Here's how the part is built. I have some questions about the finished solid (model axes, mm). A direction names the side the tool comes from. Coordinates: 2 decimals unless noted, no trailing zeros. Answer as a JSON object with one key per item and string values. Group by question number.
Q1. On a 3-axis mill with a long thin cutter (end or side, diameter ignored), from which of +Z, -Z, +X, -X, +Y, -Y can I reach the whole of each face in a straight line? I mean faces 4 (the flat face through (4, 200, 0)), 5 (the flat face through (0, 99, 4.5)). Say none if no direction works.
Q2. I need wall thicknesses on line 1 (Z direction, x = 8, y = 101.5); line 2 (Z direction, x = 3.75, y = 88.5). Which ranges of each line are inside material? Lowest first, please.
Q3. I'm going to push flat-ended pins straight in: pin 1 (0.6 mm diameter, centred on y = 59.5, z = 10, fed in from +X); pin 2 (0.6 mm diameter, centred on x = 9.5, y = 65, fed in from +Z); pin 3 (1.5 mm diameter, centred on x = -1, z = -0.5, fed in from -Y); pin 4 (2 mm diameter, centred on y = 113.5, z = 1.5, fed in from -X). Where does each tip first touch, or does it pass through?
Q4. Thinking about a two-plate mould opening in X: for faces 1 (the flat face through (10, 99, -6)), 2 (the flat face through (4, 0, 0)), 3 (the flat face through (0, 99, -4.5)), which applies, released by +X, released by -X, zero draft, split by the parting line, or undercut?
```python
from build123d import *

# Parameters (mm, degrees)
DODANIE_WYCI_GNI_CIE1_DEPTH     = 807
SCHNITT_LINEAR_AUSTRAGEN1_DEPTH = 20


with BuildPart() as part:
    # Szkic1 → Dodanie-wyciągnięcie1 (new body)
    with BuildSketch(Plane(origin=(0, 0, 0), x_dir=(1, 0, 0), z_dir=(0, 1, 0))):
        with BuildLine():
            Line((-7.06, 6), (-4.5, 3.440546933))
            Line((-4.5, 3.440546933), (-4.5, 4.5))
            Line((-4.5, 4.5), (-3.440546933, 4.5))
            Line((-3.440546933, 4.5), (-6, 7.06))
            Line((-6, 7.06), (-6, 8.5))
            Line((-6, 8.5), (-3, 8.5))
            Line((-3, 8.5), (-3, 9.5))
            Line((-3, 9.5), (-3.5, 9.5))
            Line((-3.5, 9.5), (-3.5, 10))
            Line((-3.5, 10), (-8.5, 10))
            ThreePointArc((-8.5, 10), (-9.560660172, 9.560660172), (-10, 8.5))
            Line((-10, 8.5), (-10, 3.5))
            Line((-10, 3.5), (-9.5, 3.5))
            Line((-9.5, 3.5), (-9.5, 3))
            Line((-9.5, 3), (-8.5, 3))
            Line((-8.5, 3), (-8.5, 6))
            Line((-8.5, 6), (-7.06, 6))
        make_face()
        with BuildLine():
            Line((4.5, 4.5), (4.5, 3.440546933))
            Line((4.5, 3.440546933), (7.06, 6))
            Line((7.06, 6), (8.5, 6))
            Line((8.5, 6), (8.5, 3))
            Line((8.5, 3), (9.5, 3))
            Line((9.5, 3), (9.5, 3.5))
            Line((9.5, 3.5), (10, 3.5))
            Line((10, 3.5), (10, 8.5))
            ThreePointArc((10, 8.5), (9.560660172, 9.560660172), (8.5, 10))
            Line((8.5, 10), (3.5, 10))
            Line((3.5, 10), (3.5, 9.5))
            Line((3.5, 9.5), (3, 9.5))
            Line((3, 9.5), (3, 8.5))
            Line((3, 8.5), (6, 8.5))
            Line((6, 8.5), (6, 7.06))
            Line((6, 7.06), (3.440546933, 4.5))
            Line((3.440546933, 4.5), (4.5, 4.5))
        make_face()
        Polygon((3.440546933, -4.5), (4.5, -4.5), (4.5, -3.440546933), (4.5, 3.440546933), (4.5, 4.5), (3.440546933, 4.5), (-3.440546933, 4.5), (-4.5, 4.5), (-4.5, 3.440546933), (-4.5, -3.440546933), (-4.5, -4.5), (-3.440546933, -4.5), align=None)
        with BuildLine():
            Line((-3.00520382, 1.944543648), (-1.944543648, 3.00520382))
            Line((-1.944543648, 3.00520382), (-1.271309214, 2.438498079))
            ThreePointArc((-1.271309214, 2.438498079), (0, 2.75), (1.271309214, 2.438498079))
            Line((1.271309214, 2.438498079), (1.944543648, 3.00520382))
            Line((1.944543648, 3.00520382), (3.00520382, 1.944543648))
            Line((3.00520382, 1.944543648), (2.438498079, 1.271309214))
            ThreePointArc((2.438498079, 1.271309214), (2.670989491, 0.654457899), (2.75, 0))
            ThreePointArc((2.75, 0), (2.670989491, -0.654457899), (2.438498079, -1.271309214))
            Line((2.438498079, -1.271309214), (3.00520382, -1.944543648))
            Line((3.00520382, -1.944543648), (1.944543648, -3.00520382))
            Line((1.944543648, -3.00520382), (1.271309214, -2.438498079))
            ThreePointArc((1.271309214, -2.438498079), (0, -2.75), (-1.271309214, -2.438498079))
            Line((-1.271309214, -2.438498079), (-1.944543648, -3.00520382))
            Line((-1.944543648, -3.00520382), (-3.00520382, -1.944543648))
            Line((-3.00520382, -1.944543648), (-2.438498079, -1.271309214))
            ThreePointArc((-2.438498079, -1.271309214), (-2.75, 0), (-2.438498079, 1.271309214))
            Line((-2.438498079, 1.271309214), (-3.00520382, 1.944543648))
        make_face(mode=Mode.SUBTRACT)
        with BuildLine():
            Line((-6, -7.06), (-3.440546933, -4.5))
            Line((-3.440546933, -4.5), (-4.5, -4.5))
            Line((-4.5, -4.5), (-4.5, -3.440546933))
            Line((-4.5, -3.440546933), (-7.06, -6))
            Line((-7.06, -6), (-8.5, -6))
            Line((-8.5, -6), (-8.5, -3))
            Line((-8.5, -3), (-9.5, -3))
            Line((-9.5, -3), (-9.5, -3.5))
            Line((-9.5, -3.5), (-10, -3.5))
            Line((-10, -3.5), (-10, -8.5))
            ThreePointArc((-10, -8.5), (-9.560660172, -9.560660172), (-8.5, -10))
            Line((-8.5, -10), (-3.5, -10))
            Line((-3.5, -10), (-3.5, -9.5))
            Line((-3.5, -9.5), (-3, -9.5))
            Line((-3, -9.5), (-3, -8.5))
            Line((-3, -8.5), (-6, -8.5))
            Line((-6, -8.5), (-6, -7.06))
        make_face()
        with BuildLine():
            Line((4.5, -3.440546933), (4.5, -4.5))
            Line((4.5, -4.5), (3.440546933, -4.5))
            Line((3.440546933, -4.5), (6, -7.06))
            Line((6, -7.06), (6, -8.5))
            Line((6, -8.5), (3, -8.5))
            Line((3, -8.5), (3, -9.5))
            Line((3, -9.5), (3.5, -9.5))
            Line((3.5, -9.5), (3.5, -10))
            Line((3.5, -10), (8.5, -10))
            ThreePointArc((8.5, -10), (9.560660172, -9.560660172), (10, -8.5))
            Line((10, -8.5), (10, -3.5))
            Line((10, -3.5), (9.5, -3.5))
            Line((9.5, -3.5), (9.5, -3))
            Line((9.5, -3), (8.5, -3))
            Line((8.5, -3), (8.5, -6))
            Line((8.5, -6), (7.06, -6))
            Line((7.06, -6), (4.5, -3.440546933))
        make_face()
    extrude(amount=DODANIE_WYCI_GNI_CIE1_DEPTH)

    # Skizze1 → Schnitt-Linear austragen1 (cut, symmetric)
    with BuildSketch(Plane.XY):
        Polygon((-83.496312338, 200), (63.910757592, 200), (55.14879889, 860.754768005), (-83.496312338, 858.91626029), align=None)
    extrude(amount=SCHNITT_LINEAR_AUSTRAGEN1_DEPTH, both=True, mode=Mode.SUBTRACT)


solid = part.part
```
Result set:
{
 "1": {"face 4": "+Z, -Z, +X, -X, +Y", "face 5": "+Y, -Y"},
 "2": {"line 1": "z = -10 to -6, 6 to 10", "line 2": "z = -10 to -8.5, -4.81 to 4.81, 8.5 to 10"},
 "3": {"pin 1": "stops at x = 9.4", "pin 2": "stops at z = 9.83", "pin 3": "passes through", "pin 4": "stops at x = -4.5"},
 "4": {"face 1": "released by +X", "face 2": "zero draft", "face 3": "undercut"}
}
